Source: CAD feature listing. Evaluate the final solid. Frame: model axes, mm. Round coordinates to 2 decimals unless told otherwise and drop trailing zeros. Write each loop counter-clockwise with the first axis right and the second up, starting at its lowest first coordinate (ties: lowest second). Pieces come first, ordered by that corner, then holes.
```python
from build123d import *

# Parameters (mm, degrees)
CROQUIS1_R              = 4
SALIENTE_EXTRUIR1_DEPTH = 5


with BuildPart() as part:
    # Croquis1 → Saliente-Extruir1 (new body)
    with BuildSketch(Plane.XY):
        Polygon((0, 0), (-338, 0), (-338, 25), (-388, 25), (-388, 75), (50, 75), (50, 25), (0, 25), align=None)
        with Locations((-319, 11)):
            Circle(CROQUIS1_R, mode=Mode.SUBTRACT)
        with Locations((-19, 11)):
            Circle(CROQUIS1_R, mode=Mode.SUBTRACT)
        with Locations((-169, 11)):
            Circle(CROQUIS1_R, mode=Mode.SUBTRACT)
    extrude(amount=SALIENTE_EXTRUIR1_DEPTH)


solid = part.part
```
Q1. Mould query, pull axis Y, two halves, no side actions, for faces 1 (the face through (-323, 11, 2)), 2 (the face through (-166, 38, 0)). Classes: pulls with the +Y half, pulls with the -Y half, needs draft (parallel to the pull), parting line crosses it, or undercut.
Q2. Section query B-B, the plane x = -19. Output: boundary loops of the cut face in (y, z).
Q3. Pin query (flat end, axial travel): P1, Ø2.5, axis at y = 9.5, z = 3, coming from the -X side; P2, Ø1.5, axis at x = -374.5, z = 3, coming from the -Y side; P3, Ø6.5, axis at x = -19, y = 11, coming from the +Z side. Return the tip coordinate at first contact, or that it passes through.
Q4. Line query: line 1 (Y direction, x = -19, z = 3.75); line 2 (X direction, y = 9.5, z = 3.7); line 3 (X direction, y = 5.5, z = 2.85). Output: solid intervals per line, ascending.
Q5. Section query A-A, the plane y = 11. Output: boundary loops of the cut face in (x, z).
Q6. Section query C-C, the plane z = 3.55. Output: boundary loops of the cut face in (x, y), and give its area (3 significant figures).
Filled in:
1. face 1: undercut
1. face 2: needs draft
2. outline: (0, 0) - (7, 0) - (7, 5) - (0, 5) - close; (15, 0) - (75, 0) - (75, 5) - (15, 5) - close
3. P1: stops at x = -338
3. P2: stops at y = 25
3. P3: passes through
4. line 1: y = 0 to 7, 15 to 75
4. line 2: x = -338 to -322.71, -315.29 to -172.71, -165.29 to -22.71, -15.29 to 0
4. line 3: x = -338 to 0
5. outline: (-338, 0) - (-323, 0) - (-323, 5) - (-338, 5) - close; (-315, 0) - (-173, 0) - (-173, 5) - (-315, 5) - close; (-165, 0) - (-23, 0) - (-23, 5) - (-165, 5) - close; (-15, 0) - (0, 0) - (0, 5) - (-15, 5) - close
6. outline: (-388, 25) - (-338, 25) - (-338, 0) - (0, 0) - (0, 25) - (50, 25) - (50, 75) - (-388, 75) - close; hole circle Ø8 at (-319, 11); hole circle Ø8 at (-169, 11); hole circle Ø8 at (-19, 11)
6. area: 30,200 mm2
